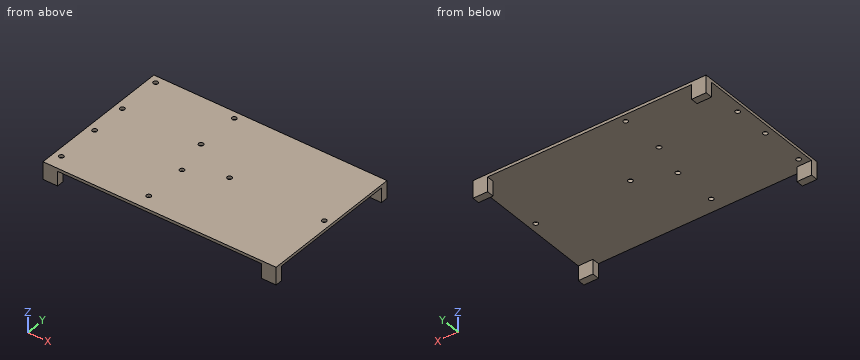
from build123d import *

# Parameters (mm, degrees)
SKETCH_1_W      = 160
SKETCH_1_H      = 100
SKETCH_1_R      = 1.6
EXTRUDE_1_DEPTH = 2
EXTRUDE_START   = -2
SKETCH_2_W      = 10
SKETCH_2_H      = 5
EXTRUDE_2_DEPTH = 10


with BuildPart() as part:
    # 草图1 → 凸台-拉伸1 (new body)
    with BuildSketch(Plane.XY):
        with Locations((19.466155548, -3.137913989)):
            Rectangle(SKETCH_1_W, SKETCH_1_H)
        with Locations((94.466155548, -3.137913989)):
            Circle(SKETCH_1_R, mode=Mode.SUBTRACT)
        with Locations((29.466155548, -3.137913989)):
            Circle(SKETCH_1_R, mode=Mode.SUBTRACT)
        with Locations((-55.533844452, -43.137913989)):
            Circle(SKETCH_1_R, mode=Mode.SUBTRACT)
        with Locations((-55.533844452, -13.137913989)):
            Circle(SKETCH_1_R, mode=Mode.SUBTRACT)
        with Locations((4.466155548, -13.137913989)):
            Circle(SKETCH_1_R, mode=Mode.SUBTRACT)
        with Locations((4.466155548, -43.137913989)):
            Circle(SKETCH_1_R, mode=Mode.SUBTRACT)
        with Locations((-55.533844452, 41.862086011)):
            Circle(SKETCH_1_R, mode=Mode.SUBTRACT)
        with Locations((-55.533844452, 11.862086011)):
            Circle(SKETCH_1_R, mode=Mode.SUBTRACT)
        with Locations((-1.533844452, 11.862086011)):
            Circle(SKETCH_1_R, mode=Mode.SUBTRACT)
        with Locations((-1.533844452, 41.862086011)):
            Circle(SKETCH_1_R, mode=Mode.SUBTRACT)
    extrude(amount=EXTRUDE_1_DEPTH)

    # 草图2 → 凸台-拉伸2 (add)
    with BuildSketch(Plane.XY.offset(2).offset(EXTRUDE_START)):
        with Locations((-55.533844452, 44.362086011)):
            Rectangle(SKETCH_2_W, SKETCH_2_H)
        with Locations((94.466155548, 44.362086011)):
            Rectangle(SKETCH_2_W, SKETCH_2_H)
        with Locations((94.466155548, -50.637913989)):
            Rectangle(SKETCH_2_W, SKETCH_2_H)
        with Locations((-55.533844452, -50.637913989)):
            Rectangle(SKETCH_2_W, SKETCH_2_H)
    extrude(amount=-EXTRUDE_2_DEPTH)


solid = part.part
Design review of the part built by this model. Coordinates are the model's own, in mm. Coordinates: 2 decimals unless noted, no trailing zeros. Order: outer loops, then holes, each group sorted by start corner. A loop starts at its lowest first (then second) coordinate and runs counter-clockwise, first axis right, second up. Notation, with made-up numbers: (-23.5, 19.25) - (33.5, 19.25) arc R13 ccw to (33.5, 38.25) - close; hole circle Ø9 at (-8.5, 30). An arc over 180 degrees is marked (long way). Put each result on its own line as item: value.
1) Take a section at C-C, the plane y = 19.5. Give the boundary of the cut face in (x, z).
Response values:
outline: (-60.53, 0) - (99.47, 0) - (99.47, 2) - (-60.53, 2) - close
2) Take a section at B-B, the plane x = 82. Give the boundary of the cut face in (y, z).
Response values:
outline: (-53.14, 0) - (46.86, 0) - (46.86, 2) - (-53.14, 2) - close
3) Insertion check: P1, Ø4, axis at x = -1.53, y = 41.86, coming from the -Z side. The pin has a flat end and moves straight along its axis. Give the tip position at first contact, or say it passes through.
Response values:
P1: stops at z = 0
4) Take a section at A-A, the plane z = -4.5. Give the boundary of the cut face in (x, y).
Response values:
outline: (-60.53, -53.14) - (-50.53, -53.14) - (-50.53, -48.14) - (-60.53, -48.14) - close; (-60.53, 41.86) - (-50.53, 41.86) - (-50.53, 46.86) - (-60.53, 46.86) - close; (89.47, -53.14) - (99.47, -53.14) - (99.47, -48.14) - (89.47, -48.14) - close; (89.47, 41.86) - (99.47, 41.86) - (99.47, 46.86) - (89.47, 46.86) - close
5) Wall thickness on L1, parallel to Z at x = 24, y = -43; L2, parallel to Y at x = 92.5, z = -8: over which ranges is each line inside the solid? List them lowest first. Write a range as from..to.
Response values:
L1: z = 0..2
L2: y = -53.14..-48.14, 41.86..46.86
